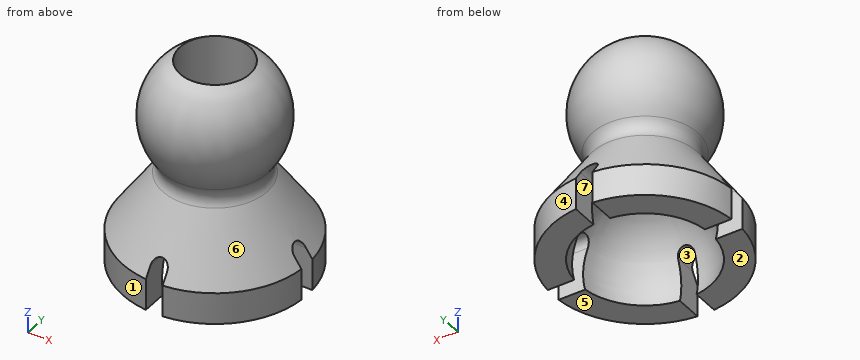
```python
from build123d import *

# Parameters (mm, degrees)
F2_R     = 4.208015
F3_DEPTH = 25
F5_DEPTH = 12.5
F7_DEPTH = 12.5


with BuildPart() as f1:
    # F0 (on Front) → F1 (revolve)
    with BuildSketch(Plane.XZ):
        with BuildLine():
            Line((0, 19.985304), (0, 4.185304))
            ThreePointArc((0, 4.185304), (0.592961, 4.207589), (1.182577, 4.274317))
            ThreePointArc((1.182577, 4.274317), (6.796412, 0.728365), (7.926577, -5.814696))
            Line((7.926577, -5.814696), (11.100425, -5.814696))
            Line((11.100425, -5.814696), (11.100425, -2.018886))
            Line((11.100425, -2.018886), (6.278364, 5.02771))
            ThreePointArc((6.278364, 5.02771), (5.92934, 6.19907), (6.327103, 7.354789))
            ThreePointArc((6.327103, 7.354789), (7.063323, 15.62359), (0, 19.985304))
        make_face()
    revolve(axis=Axis((0, 0, -0.814696), (0, 0, -1)))

    # F2 (on Top) → F3 (cut, symmetric)
    with BuildSketch(Plane.XY):
        Circle(F2_R)
    extrude(amount=F3_DEPTH, both=True, mode=Mode.SUBTRACT)

    # F4 (on Right) → F5 (cut, symmetric)
    with BuildSketch(Plane.YZ):
        with BuildLine():
            Line((-1, -5.814696), (1, -5.814696))
            Line((1, -5.814696), (1, -0.914696))
            ThreePointArc((1, -0.914696), (0.052562, 0.186553), (-1, -0.814696))
            Line((-1, -0.814696), (-1, -5.814696))
        make_face()
    extrude(amount=F5_DEPTH, both=True, mode=Mode.SUBTRACT)

    # F6 (on Front) → F7 (cut, symmetric)
    with BuildSketch(Plane.XZ):
        with BuildLine():
            Line((-1, -0.814696), (-1, -5.814696))
            Line((-1, -5.814696), (1, -5.814696))
            Line((1, -5.814696), (1, -0.814696))
            ThreePointArc((1, -0.814696), (0, 0.185304), (-1, -0.814696))
        make_face()
    extrude(amount=F7_DEPTH, both=True, mode=Mode.SUBTRACT)


solid = f1.part
```
Source: CAD feature listing. Evaluate the final solid. Frame: model axes, mm. Face numbers are marked on the shaded views. A direction names the side the tool comes from. Give positions to 0.01 mm unless a question says otherwise; leave off trailing zeros. Put each result on its own line as item: value. Start each with the question number.
1) Reachability of the marked faces 5, 6 and 7 from +Z, -Z, +X, -X, +Y, -Y: full face, straight path, thin tool, end or side. Return the list, or none.
2) Material intervals for probe 1 along Y at (x, z) = (0, 15.75); probe 2 along Y at (x, z) = (0, 15); probe 3 along Z at (x, y) = (6.5, -2), sorted ascending.
3) Draft query along X for the marked faces 1, 2, 3 and 4. Return one class per face: released by +X, released by -X, zero draft, split by the parting line, or undercut.
4) Contact query for flat-ended pins moving along their axis: P1, Ø4, axis at x = 6.5, z = 0.5, coming from the +Y side; P2, Ø3, axis at x = -6.5, z = 11, coming from the +Y side; P3, Ø1.1, axis at y = -9.5, z = -4.5, coming from the +X side. Output: stop coordinate, or through.
Results are:
1. face 5: -Z, +X, -X, +Y, -Y
1. face 6: none
1. face 7: -Z, +Y, -Y
2. probe 1: y = -7 to -4.21, 4.21 to 7
2. probe 2: y = -7.34 to -4.21, 4.21 to 7.34
2. probe 3: z = 0.72 to 4.26, 8.07 to 16.11
3. face 1: released by -X
3. face 2: zero draft
3. face 3: undercut
3. face 4: released by +X
4. P1: stops at y = 9.03
4. P2: stops at y = 6.04
4. P3: stops at x = 6.57
